Build history of the part. All positions in model axes, mm. Round coordinates to 2 decimals unless told otherwise and drop trailing zeros. Write each loop counter-clockwise with the first axis right and the second up, starting at its lowest first coordinate (ties: lowest second). Pieces come first, ordered by that corner, then holes.
1) Saw through at A-A (z = -27). Write the cut outline in (x, y) (3 decimals), plus the area to 3 significant figures.
2) Saw through at B-B (y = -7). Write the cut outline in (x, z), plus the area to 3 significant figures.
3) Wall check: probe 1 along X at (y, z) = (17.5, 1) (3 decimals); probe 2 along Y at (x, z) = (-1, 23); probe 3 along X at (y, z) = (-5.5, 26). Give the ranges that are in metal, low to high.
4) Saw through at C-C (x = -11). Write the cut outline in (y, z).
5) Flat gauge pins, fed straight in: pin 1 (19 mm diameter, centred on y = 25, z = 6, fed in from +X) (3 decimals); pin 2 (4 mm diameter, centred on x = 6.5, z = 11, fed in from -Y); pin 3 (1 mm diameter, centred on y = 31, z = 7, fed in from -X) (3 decimals). Where does each tip first touch, or does it go through?
Autodesk Inventor part; units mm, degrees
ref_plane "YZ Plane" through (0, 0, 0) normal (1, 0, 0) x (0, 1, 0)
ref_plane "XZ Plane" through (0, 0, 0) normal (0, 1, 0) x (-1, 0, 0)
ref_plane "XY Plane" through (0, 0, 0) normal (0, 0, 1) x (1, 0, 0)
sketch "Sketch1" plane through (0, 0, 0) normal (0, 0, 1) x (1, 0, 0)
  circle A0 centre (0, 0) radius 17.705
  circle A1 centre (0, 0) radius 15
  circle A2 centre (0, 15) radius 0.75
  circle A3 centre (-10.6066, 10.6066) radius 0.75
  circle A4 centre (0, 0) radius 15
  circle A5 centre (-15, 0) radius 0.75
  circle A6 centre (0, 0) radius 15
  circle A7 centre (-10.6066, -10.6066) radius 0.75
  circle A8 centre (0, 0) radius 15
  circle A9 centre (0, -15) radius 0.75
  circle A10 centre (0, 0) radius 15
  circle A11 centre (10.6066, -10.6066) radius 0.75
  circle A12 centre (0, 0) radius 15
  circle A13 centre (15, 0) radius 0.75
  circle A14 centre (0, 0) radius 15
  circle A15 centre (10.6066, 10.6066) radius 0.75
  circle A16 centre (0, 0) radius 15
  line L0 (-20.705, 38) -> (20.705, 38)
  arc A17 (0, -20.705) -> (20.705, 0) centre (0.7179, -0.7179) ccw
  arc A18 (-20.705, 0) -> (0, -20.705) centre (-0.7179, -0.7179) ccw
  line L1 (-20.705, 0) -> (-20.705, 38)
  line L2 (20.705, 38) -> (20.705, 0)
  dimension "d1" = 30
  dimension "d0" = 35.41
  dimension "d2" = 1.5
  dimension "d5" = 360
  dimension "d10" = 38
  dimension "d11" = 20
  dimension "d12" = 20
  dimension "d15" = 58.705
sketch "Sketch2" plane through (0, 0, 0) normal (0, 0, 1) x (1, 0, 0)
  point P0 (0, 0)
sketch "Sketch3" plane through (0, 0, 0) normal (0, 0, 1) x (1, 0, 0)
  point P0 (0, 0)
sketch "Sketch4" plane through (0, 0, 0) normal (0, 0, 1) x (1, 0, 0)
  point P0 (0, 0)
extrude "Extrusion1" add sketch "Sketch1" along normal mid plane 64 contours A0 | A1 A13 | A1 A13 | A13 A1 A11 A9 A7 A5 A3 A2 A15 | A15 A1 | A1 A15 | A11 A1 | A1 A11 | A2 A1 | A1 A2 | A9 A1 | A1 A9 | A3 A1 | A1 A3 | A7 A1 | A1 A7 | A5 A1 | A1 A5 | L0 L2 A17 A18 L1
properties part number "Horn"
Evaluation:
1. outline: (-20.705, 0) arc R20 ccw to (0, -20.705) arc R20 ccw to (20.705, 0) - (20.705, 38) - (-20.705, 38) - close
1. area: 2,260 mm2
2. outline: (-19.71, -32) - (19.71, -32) - (19.71, 32) - (-19.71, 32) - close
2. area: 2,520 mm2
3. probe 1: x = -20.705 to 20.705
3. probe 2: y = -20.72 to 38
3. probe 3: x = -20.14 to 20.14
4. outline: (-17.87, -32) - (38, -32) - (38, 32) - (-17.87, 32) - close
5. pin 1: stops at x = 20.705
5. pin 2: stops at y = -20.36
5. pin 3: stops at x = -20.705
